Part model, mm, in its own coordinate system. A direction names the side the tool comes from. Give positions to 0.01 mm unless a question says otherwise; leave off trailing zeros. Order: outer loops, then holes, each group sorted by start corner. A loop starts at its lowest first (then second) coordinate and runs counter-clockwise, first axis right, second up. Notation, with made-up numbers: (-25.75, 54) - (4.25, 54) arc R26 cw to (4.25, 78) - close; hole circle Ø8 at (69, 24.5). An arc over 180 degrees is marked (long way). One line per item, written item: value.
Autodesk Inventor part; units mm, degrees
ref_plane "YZ Plane" through (0, 0, 0) normal (1, 0, 0) x (0, 1, 0)
ref_plane "XZ Plane" through (0, 0, 0) normal (0, 1, 0) x (-1, 0, 0)
ref_plane "XY Plane" through (0, 0, 0) normal (0, 0, 1) x (1, 0, 0)
sketch "Sketch1" plane through (0, 0, 0) normal (1, 0, 0) x (0, 1, 0)
  line L0 (0, 0) -> (0, -2.1848) construction
  line L1 (0, 0) -> (4, 0) construction
  line L2 (4, 0) -> (4, -1.75)
  line L3 (4, -1.75) -> (4.25, -1.75)
  line L4 (4.25, -1.75) -> (4.25, -1.65)
  line L5 (4.25, -1.65) -> (5.75, -1.65)
  line L6 (5.75, -1.65) -> (5.75, -1.75)
  line L7 (5.75, -1.75) -> (6, -1.75)
  line L8 (6, -1.75) -> (6, 0)
  line L9 (6, 0) -> (4, 0) construction
  line L10 (4, 0) -> (4, 1.75)
  line L11 (4, 1.75) -> (4.25, 1.75)
  line L12 (4.25, 1.75) -> (4.25, 1.65)
  line L13 (4.25, 1.65) -> (5.75, 1.65)
  line L14 (5.75, 1.65) -> (5.75, 1.75)
  line L15 (5.75, 1.75) -> (6, 1.75)
  line L16 (6, 1.75) -> (6, 0)
  dimension "d0" = 4
  dimension "d1" = 6
  dimension "d2" = 0.1
  dimension "d3" = 1.5
  dimension "d6" = 3.5
revolve "Revolution1" add sketch "Sketch1" angle 360 about axis through (0, 0, 0) along (0, 0, -1)
properties part number "MR128 bearing"
1) Drill centre lines: line 1 along X through (y, z) = (0, 1.7); line 2 along X through (y, z) = (0, 0.5); line 3 along Z through (x, y) = (1.25, 5). Where is each one in solid material? Low to high. Write a range as from..to.
Outcome:
line 1: x = -6..-5.75, -4.25..-4, 4..4.25, 5.75..6
line 2: x = -6..-4, 4..6
line 3: z = -1.65..1.65
2) Which spindle directions (+Z, -Z, +X, -X, +Y, -Y) get a long thin tool onto all of the face, cutting with end or side? Do faces 1 (the cylindrical face through (-3.905, -0.867, -0.024)), 2 (the flat face through (-4, -2, 1.65)). Say none if no direction does.
Outcome:
face 1: +Z, -Z
face 2: +Z
3) Pin check, flat tips, straight feed: pin 1 (1 mm diameter, centred on y = -1, z = -1, fed in from +X); pin 2 (1 mm diameter, centred on x = -2, z = 1.5, fed in from +Y); pin 3 (1 mm diameter, centred on x = -4.5, z = 1, fed in from -Y). Stop position of each tip, or through.
Outcome:
pin 1: stops at x = 5.98
pin 2: stops at y = 5.81
pin 3: stops at y = -4.47
4) Cut at A-A, the plane y = 0. Give the cut face in (x, z).
Outcome:
outline: (-6, -1.75) - (-5.75, -1.75) - (-5.75, -1.65) - (-4.25, -1.65) - (-4.25, -1.75) - (-4, -1.75) - (-4, 1.75) - (-4.25, 1.75) - (-4.25, 1.65) - (-5.75, 1.65) - (-5.75, 1.75) - (-6, 1.75) - close; (4, -1.75) - (4.25, -1.75) - (4.25, -1.65) - (5.75, -1.65) - (5.75, -1.75) - (6, -1.75) - (6, 1.75) - (5.75, 1.75) - (5.75, 1.65) - (4.25, 1.65) - (4.25, 1.75) - (4, 1.75) - close
5) Mould opens along Y. For faces 3 (the cylindrical face through (0, -6, 0)), 4 (the flat face through (-4, -2, -1.65)) say: released by +Y, released by -Y, zero draft, split by the parting line, or undercut.
Outcome:
face 3: split by the parting line
face 4: undercut
6) Cut at C-C, the plane z = 0.65. Give the cut face in (x, y).
Outcome:
outline: circle Ø12 at (0, 0); hole circle Ø8 at (0, 0)
